Work out the finished part from the listing and answer in its coordinate system (mm). Round coordinates to 2 decimals unless told otherwise and drop trailing zeros. Order: outer loops, then holes, each group sorted by start corner. A loop starts at its lowest first (then second) coordinate and runs counter-clockwise, first axis right, second up. Notation, with made-up numbers: (1.5, -24.5) - (42.5, -24.5) arc R18 cw to (42.5, 9.5) - close; hole circle Ø10 at (4.5, -10). An arc over 180 degrees is marked (long way). Answer in a Markdown table with one row per item.
from build123d import *

# Parameters (mm, degrees)
SKETCH1_W           = 30
SKETCH1_H           = 160
BOSS_EXTRUDE1_DEPTH = 5.2
CUT_EXTRUDE1_DEPTH  = 10


with BuildPart() as part:
    # Sketch1 → Boss-Extrude1 (new body)
    with BuildSketch(Plane(origin=(0, 0, 0), x_dir=(1, 0, 0), z_dir=(0, 1, 0))):
        with Locations((15, 80)):
            Rectangle(SKETCH1_W, SKETCH1_H)
    extrude(amount=BOSS_EXTRUDE1_DEPTH)

    # Sketch2 → Cut-Extrude1 (cut)
    with BuildSketch(Plane(origin=(0, 5.2, 0), x_dir=(1, 0, 0), z_dir=(0, 1, 0))):
        Polygon((30, 131.642135624), (22.221825407, 139.420310217), (30, 147.19848481), align=None)
        Polygon((30, 19.142135624), (22.928932188, 12.071067812), (30, 5), align=None)
    extrude(amount=-CUT_EXTRUDE1_DEPTH, mode=Mode.SUBTRACT)


solid = part.part
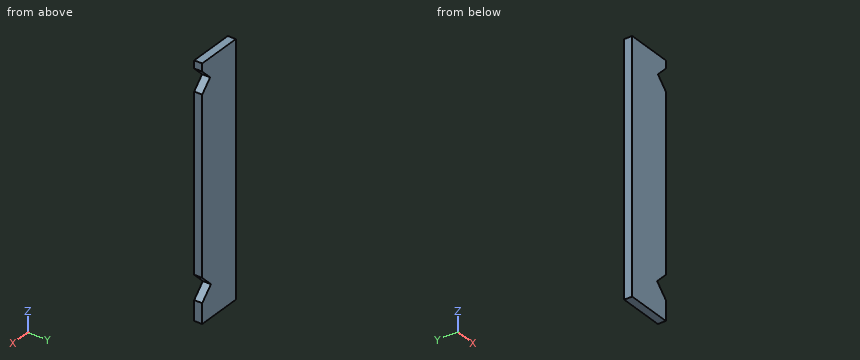
1) This flat-tipped pin is pushed along its axis until it touches: pin 1 (3 mm diameter, centred on y = 2.5, z = -108.5, fed in from -X). Where does it stop, or does it pass through?
Filled in:
| item | result |
|---|---|
| pin 1 | stops at x = 0 |
2) Find section A-A, the plane y = 3.6. Give the vertices of the cut face in (x, z).
Filled in:
| item | result |
|---|---|
| outline | (0, -160) - (30, -160) - (30, -147.2) - (22.22, -139.42) - (30, -131.64) - (30, -19.14) - (22.93, -12.07) - (30, -5) - (30, 0) - (0, 0) - close |
3) Find section B-B, the plane x = 27.5. Give the vertices of the cut face in (y, z), then the cut area to 3 significant figures.
Filled in:
| item | result |
|---|---|
| outline | (0, -160) - (5.2, -160) - (5.2, -144.7) - (0, -144.7) - close; (0, -134.14) - (5.2, -134.14) - (5.2, -16.64) - (0, -16.64) - close; (0, -7.5) - (5.2, -7.5) - (5.2, 0) - (0, 0) - close |
| area | 730 mm^2 |
4) Find section C-C, the plane z = -141.5. Give the vertices of the cut face in (x, y).
Filled in:
| item | result |
|---|---|
| outline | (0, 0) - (24.3, 0) - (24.3, 5.2) - (0, 5.2) - close |
5) Find the intervals of material crossed by probe 1 along Z at (x, y) = (24, 1.6); probe 2 along Z at (x, y) = (25, 3.4); probe 3 along X at (y, z) = (3.6, -143.5), in increasing order. Write a range as from..to.
Filled in:
| item | result |
|---|---|
| probe 1 | z = -160..-141.2, -137.64..-13.14, -11..0 |
| probe 2 | z = -160..-142.2, -136.64..-14.14, -10..0 |
| probe 3 | x = 0..26.3 |
